Geometry check sheet. Reference: the model listing, model coordinates, mm. A direction names the side the tool comes from. Give positions to 0.01 mm unless a question says otherwise; leave off trailing zeros. Loops run counter-clockwise (first coordinate to the right, second up) from the corner with the lowest first, then second, coordinate; pieces in that order, holes last. Notation, with made-up numbers: (28, 53.25) -> (35, 53.25) arc R8 cw to (35, 57.25) -> close; hole circle Ø1 at (71.5, -34.75). An arc over 180 degrees is marked (long way). Write item = value, one per line. Start each with the question number.
```python
from build123d import *

# Parameters (mm, degrees)
F0_W     = 57.15
F0_H     = 31.75
F1_DEPTH = 3.175
F2_W     = 49.392026
F2_H     = 24.930672
F3_DEPTH = 50.8
F4_W     = 43.211122
F4_H     = 41.259654
F5_DEPTH = 12.7
F6_SIZE  = 1.27
F7_R     = 0.508


with BuildPart() as f1:
    # F0 (on Front) → F1 (new body, symmetric)
    with BuildSketch(Plane.XZ):
        Rectangle(F0_W, F0_H)
    extrude(amount=F1_DEPTH, both=True)

    # F2 (on Front) → F3 (join)
    with BuildSketch(Plane.XZ):
        Rectangle(F2_W, F2_H)
    extrude(amount=-F3_DEPTH)

    # F4 (on face) → F5 (cut)
    with BuildSketch(Plane.XY.offset(12.465336)):
        with Locations((0, 26.623629)):
            Rectangle(F4_W, F4_H)
    extrude(amount=-F5_DEPTH, mode=Mode.SUBTRACT)

    # F6
    f6_edges = [f1.edges().sort_by_distance(p)[0] for p in [
        (0, -3.175, -15.875),
        (-28.575, -3.175, 0),
        (28.575, -3.175, 0),
        (0, -3.175, 15.875),
    ]]
    chamfer(f6_edges, length=F6_SIZE)

    # F7
    f7_edges = [f1.edges().sort_by_distance(p)[0] for p in [
        (0, -3.175, -14.605),
        (-27.305, -3.175, 0),
        (27.305, -3.175, 0),
        (0, -3.175, 14.605),
    ]]
    fillet(f7_edges, radius=F7_R)


solid = f1.part
```
1) Draft check along Y on faces 4 (the flat face through (0, 5, 12.465)), 5 (the flat face through (21.606, 26, 6)), 6 (the flat face through (0, -3.175, 0)). Enter one of: released by +Y, released by -Y, zero draft, split by the parting line, or undercut.
2) Section check D-D (y = 31). Enter the section's corners in (x, z), plus the area to 3 significant figures.
3) Section check C-C (z = -9). Enter the section's corners in (x, y) (3 decimals).
4) Section check A-A (z = 9). Enter the section's corners in (x, y) (3 decimals).
5) Section check B-B (x = 25.5). Enter the section's corners in (y, z) (3 decimals), plus the area to 3 significant figures.
6) Tool access check on faces 1 (the flat face through (-24.696, 27, 0)), 2 (the flat face through (0, 47.253, 6)), 3 (the flat face through (0, 27, -12.465)). Record the directions out of +Z, -Z, +X, -X, +Y, -Y that give a thin tool (end or side, any length) a straight path to the whole face; none if there is none.
7) Depth check by flat-ended pin: pin 1 Ø3 at (x, y) = (11, 32.5) entering from -Z; pin 2 Ø14.5 at (x, y) = (-5, 19.5) entering from +Z; pin 3 Ø5 at (y, z) = (14.5, 11.5) entering from -X; pin 4 Ø5 at (x, y) = (-4.5, 3.5) entering from +Z (3 decimals). Enter the tip coordinate at first touch or a pass-through.
8) Thickness scan on line 1 (X direction, y = 32, z = 6.5); line 2 (Y direction, x = 21, z = 7.5) (3 decimals); line 3 (X direction, y = 12.5, z = -4.5). Record the ranges inside material, lowest first.
Check result:
q1.face_4 = zero draft
q1.face_5 = undercut
q1.face_6 = released by -Y
q2.outline = (-24.7, -12.47) -> (24.7, -12.47) -> (24.7, 12.47) -> (21.61, 12.47) -> (21.61, -0.23) -> (-21.61, -0.23) -> (-21.61, 12.47) -> (-24.7, 12.47) -> close
q2.area = 683 mm2
q3.outline = (-28.575, -1.905) -> (-27.454, -3.026) arc R0.508 ccw to (-27.095, -3.175) -> (27.095, -3.175) arc R0.508 ccw to (27.454, -3.026) -> (28.575, -1.905) -> (28.575, 3.175) -> (24.696, 3.175) -> (24.696, 50.8) -> (-24.696, 50.8) -> (-24.696, 3.175) -> (-28.575, 3.175) -> close
q4.outline = (-28.575, -1.905) -> (-27.454, -3.026) arc R0.508 ccw to (-27.095, -3.175) -> (27.095, -3.175) arc R0.508 ccw to (27.454, -3.026) -> (28.575, -1.905) -> (28.575, 3.175) -> (24.696, 3.175) -> (24.696, 50.8) -> (-24.696, 50.8) -> (-24.696, 3.175) -> (-28.575, 3.175) -> close; hole (-21.606, 5.994) -> (21.606, 5.994) -> (21.606, 47.253) -> (-21.606, 47.253) -> close
q5.outline = (-3.175, -14.395) arc R0.508 ccw to (-3.026, -14.754) -> (-1.905, -15.875) -> (3.175, -15.875) -> (3.175, 15.875) -> (-1.905, 15.875) -> (-3.026, 14.754) arc R0.508 ccw to (-3.175, 14.395) -> close
q5.area = 200 mm2
q6.face_1 = +Z, -Z, -X, +Y
q6.face_2 = +Z
q6.face_3 = -Z, +X, -X, +Y
q7.pin_1 = -12.47
q7.pin_2 = -0.23
q7.pin_3 = -24.7
q7.pin_4 = 15.875
q8.line_1 = -24.7 to -21.61, 21.61 to 24.7
q8.line_2 = -3.175 to 5.994, 47.253 to 50.8
q8.line_3 = -24.7 to 24.7
